Could you check a few things on this model? Use its own coordinates, in mm. A direction names the side the tool comes from. Round coordinates to 2 decimals unless told otherwise and drop trailing zeros. Loops run counter-clockwise (first coordinate to the right, second up) from the corner with the lowest first, then second, coordinate; pieces in that order, holes last. Notation, with made-up numbers: (-32, 14) - (18, 14) arc R13 ccw to (18, 20) - close; hole circle Ø5 at (27, 44.5). An arc over 180 degrees is marked (long way). Put each result on its own line as item: value. Start each with the question number.
from build123d import *

# Parameters (mm, degrees)
SKETCH1_W           = 86.36
SKETCH1_H           = 108.458
SKETCH1_R           = 3
SKETCH1_R_2         = 3.2
SKETCH1_W_2         = 14.993601523
SKETCH1_H_2         = 4.4218346
SKETCH1_W_3         = 14.993536873
SKETCH1_H_3         = 5.57414232
SKETCH1_W_4         = 3.620082636
SKETCH1_H_4         = 27.166637837
SKETCH1_W_5         = 2.05031229
SKETCH1_H_5         = 29.189687669
BOSS_EXTRUDE1_DEPTH = 1.778
SKETCH1_4_R         = 3.2
SKETCH1_4_R_2       = 1.6
BOSS_EXTRUDE2_DEPTH = 5.715
SKETCH1_5_W         = 14.993601523
SKETCH1_5_H         = 4.4218346
SKETCH1_5_W_2       = 14.993536873
SKETCH1_5_H_2       = 5.57414232
SKETCH1_5_W_3       = 3.620082636
SKETCH1_5_H_3       = 27.166637837
SKETCH1_5_W_4       = 2.05031229
SKETCH1_5_H_4       = 29.189687669
BOSS_EXTRUDE3_DEPTH = 33.02


with BuildPart() as part:
    # Sketch1 → Boss-Extrude1 (new body)
    with BuildSketch(Plane(origin=(0, 0, 0), x_dir=(1, 0, 0), z_dir=(0, 1, 0))):
        with Locations((-2.221461279, 28.121370378)):
            Rectangle(SKETCH1_W, SKETCH1_H)
        with Locations(Location((-34.610055164, 70.822519266, 0), (0, 0, 270))):
            Circle(SKETCH1_R, mode=Mode.SUBTRACT)
        with Locations(Location((21.943044836, 70.822519266, 0), (0, 0, 270))):
            Circle(SKETCH1_R, mode=Mode.SUBTRACT)
        with Locations(Location((-34.610055164, 34.576719266, 0), (0, 0, 270))):
            Circle(SKETCH1_R, mode=Mode.SUBTRACT)
        with Locations(Location((21.943044836, 34.576719266, 0), (0, 0, 270))):
            Circle(SKETCH1_R, mode=Mode.SUBTRACT)
        with Locations(Location((-36.36256187, 22.219519164, 0), (0, 0, 270))):
            Circle(SKETCH1_R_2, mode=Mode.SUBTRACT)
        with Locations(Location((28.15343813, 22.219519164, 0), (0, 0, 270))):
            Circle(SKETCH1_R_2, mode=Mode.SUBTRACT)
        with Locations(Location((-36.36256187, -17.150480836, 0), (0, 0, 270))):
            Circle(SKETCH1_R_2, mode=Mode.SUBTRACT)
        with Locations(Location((28.15343813, -17.150480836, 0), (0, 0, 270))):
            Circle(SKETCH1_R_2, mode=Mode.SUBTRACT)
        with Locations((-36.756055824, 80.051074351)):
            Rectangle(SKETCH1_W_2, SKETCH1_H_2, mode=Mode.SUBTRACT)
        with Locations((32.441242145, 78.064404156)):
            Rectangle(SKETCH1_W_3, SKETCH1_H_3, mode=Mode.SUBTRACT)
        with Locations((37.551401815, -1.544112086)):
            Rectangle(SKETCH1_W_4, SKETCH1_H_4, mode=Mode.SUBTRACT)
        with Locations((-43.291771042, -2.555637001)):
            Rectangle(SKETCH1_W_5, SKETCH1_H_5, mode=Mode.SUBTRACT)
    extrude(amount=BOSS_EXTRUDE1_DEPTH)

    # Sketch1_4 → Boss-Extrude2 (add)
    # profile 1 of 4: a face of its own
    with BuildSketch(Plane(origin=(0, 0, 0), x_dir=(1, 0, 0), z_dir=(0, 1, 0))):
        with Locations(Location((-36.36256187, -17.150480836, 0), (0, 0, 270))):
            Circle(SKETCH1_4_R)
        with Locations(Location((-36.36256187, -17.150480836, 0), (0, 0, 270))):
            Circle(SKETCH1_4_R_2, mode=Mode.SUBTRACT)
    # profile 2 of 4: a face of its own
    with BuildSketch(Plane(origin=(0, 0, 0), x_dir=(1, 0, 0), z_dir=(0, 1, 0))):
        with Locations(Location((28.15343813, -17.150480836, 0), (0, 0, 270))):
            Circle(SKETCH1_4_R)
        with Locations(Location((28.15343813, -17.150480836, 0), (0, 0, 270))):
            Circle(SKETCH1_4_R_2, mode=Mode.SUBTRACT)
    # profile 3 of 4: a face of its own
    with BuildSketch(Plane(origin=(0, 0, 0), x_dir=(1, 0, 0), z_dir=(0, 1, 0))):
        with Locations(Location((28.15343813, 22.219519164, 0), (0, 0, 270))):
            Circle(SKETCH1_4_R)
        with Locations(Location((28.15343813, 22.219519164, 0), (0, 0, 270))):
            Circle(SKETCH1_4_R_2, mode=Mode.SUBTRACT)
    # profile 4 of 4: a face of its own
    with BuildSketch(Plane(origin=(0, 0, 0), x_dir=(1, 0, 0), z_dir=(0, 1, 0))):
        with Locations(Location((-36.36256187, 22.219519164, 0), (0, 0, 270))):
            Circle(SKETCH1_4_R)
        with Locations(Location((-36.36256187, 22.219519164, 0), (0, 0, 270))):
            Circle(SKETCH1_4_R_2, mode=Mode.SUBTRACT)
    extrude(amount=BOSS_EXTRUDE2_DEPTH)

    # Sketch1_5 → Boss-Extrude3 (add)
    with BuildSketch(Plane(origin=(0, 0, 0), x_dir=(1, 0, 0), z_dir=(0, 1, 0))):
        with Locations((-36.756055824, 80.051074351)):
            Rectangle(SKETCH1_5_W, SKETCH1_5_H)
        with Locations((32.441242145, 78.064404156)):
            Rectangle(SKETCH1_5_W_2, SKETCH1_5_H_2)
        with Locations((37.551401815, -1.544112086)):
            Rectangle(SKETCH1_5_W_3, SKETCH1_5_H_3)
        with Locations((-43.291771042, -2.555637001)):
            Rectangle(SKETCH1_5_W_4, SKETCH1_5_H_4)
    extrude(amount=BOSS_EXTRUDE3_DEPTH)


solid = part.part
Item 1: On a 3-axis mill with a long thin cutter (end or side, diameter ignored), from which of +Z, -Z, +X, -X, +Y, -Y can I reach the whole of each face in a straight line? I mean faces 1 (the face through (35.741, 17, 2)), 2 (the face through (-37, 17, -77.84)), 3 (the face through (38, 17, 15.127)), 4 (the face through (30.85, 3.72, 18.87)). Say none if no direction works.
Item 2: I need wall thicknesses on line 1 (X direction, y = 4, z = 10); line 2 (Z direction, x = 36, y = 28); line 3 (X direction, y = 5, z = 17.5). Which ranges of each line are inside material? Lowest first, please. Write a range as from..to.
Item 3: Thinking about a two-plate mould opening in Z: for faces 5 (the face through (-35, 5.715, 16)), 6 (the face through (-37.925, 2.817, 16.804)), 7 (the face through (32, 17, -80.851)), which applies, released by +Z, released by -Z, zero draft, split by the parting line, or undercut?
Item 4: Will these pins go through, and if not, where does the flat tip stop? P1, Ø3, axis at x = -35.5, z = 17, coming from the +Y side (3 decimals); P2, Ø1.7, axis at y = 14.5, z = -77.5, coming from the +X side; P3, Ø16.5, axis at x = -38, y = 22, coming from the -Z side.
Item 5: Suppose I cut it at D-D, the plane x = -1.5. List the corners of the cut face in (y, z) for me, then the cut area to 3 significant figures.
Item 6: Suppose I cut it at A-A, the plane y = 21. List the corners of the cut face in (x, z) for me.
Item 7: Suppose I cut it at B-B, the plane z = -70. List the corners of the cut face in (x, y) for me, then the cut area to 3 significant figures.
Item 8: Suppose I cut it at C-C, the plane y = 3. Count the separate pieces of the cut face and the enclosed holes in it, then the cut area to 3 significant figures.
Numbers:
1. face 1: +Z, +Y
1. face 2: -X, +Y
1. face 3: +Z, +X, +Y
1. face 4: +Y
2. line 1: -44.32..-42.27, 35.74..39.36
2. line 2: -80.85..-75.28, -12.04..15.13
2. line 3: -39.54..-37.92, -34.8..-33.18, 24.97..26.59, 29.71..31.33
3. face 5: zero draft
3. face 6: undercut
3. face 7: released by -Z
4. P1: y = 5.715
4. P2: x = 39.94
4. P3: z = -82.26
5. outline: (0, -82.35) - (1.78, -82.35) - (1.78, 26.11) - (0, 26.11) - close
5. area: 193 mm^2
6. outline: (-44.32, -12.04) - (-42.27, -12.04) - (-42.27, 17.15) - (-44.32, 17.15) - close; (-44.25, -82.26) - (-29.26, -82.26) - (-29.26, -77.84) - (-44.25, -77.84) - close; (24.94, -80.85) - (39.94, -80.85) - (39.94, -75.28) - (24.94, -75.28) - close; (35.74, -12.04) - (39.36, -12.04) - (39.36, 15.13) - (35.74, 15.13) - close
7. outline: (-45.4, 0) - (-37.5, 0) - (-37.5, 1.78) - (-45.4, 1.78) - close; (-31.73, 0) - (19.06, 0) - (19.06, 1.78) - (-31.73, 1.78) - close; (24.83, 0) - (40.96, 0) - (40.96, 1.78) - (24.83, 1.78) - close
7. area: 133 mm^2
8. separate pieces: 8
8. enclosed holes: 4
8. area: 405 mm^2
